```python
from build123d import *

# Parameters (mm, degrees)
BOSS_EXTRUDE1_DEPTH = 57.15
SKETCH2_W           = 44.45
SKETCH2_H           = 66.04
CUT_EXTRUDE1_DEPTH  = 57.15
SKETCH6_R           = 4.7625
CUT_EXTRUDE3_DEPTH  = 3.175
SKETCH8_R           = 0.79375
CUT_EXTRUDE4_DEPTH  = 58.15


with BuildPart() as part:
    # Sketch1 → Boss-Extrude1 (new body)
    with BuildSketch(Plane.XY):
        with BuildLine():
            Line((-15.24, 76.2), (-15.24, -76.2))
            ThreePointArc((-15.24, -76.2), (0, -91.44), (15.24, -76.2))
            Line((15.24, -76.2), (15.24, 76.2))
            ThreePointArc((15.24, 76.2), (0, 91.44), (-15.24, 76.2))
        make_face()
    extrude(amount=BOSS_EXTRUDE1_DEPTH)

    # Sketch2 → Cut-Extrude1 (cut)
    with BuildSketch(Plane(origin=(15.24, 0, 0), x_dir=(0, 0, -1), z_dir=(1, 0, 0))):
        with Locations((-28.575, 58.42)):
            Rectangle(SKETCH2_W, SKETCH2_H)
    cut_extrude1 = extrude(amount=-CUT_EXTRUDE1_DEPTH, mode=Mode.SUBTRACT)

    # Sketch6 → Cut-Extrude3 (cut)
    with BuildSketch(Plane.XY.offset(6.35)):
        with Locations((0, 76.2)):
            Circle(SKETCH6_R)
    cut_extrude3 = extrude(amount=-CUT_EXTRUDE3_DEPTH, mode=Mode.SUBTRACT)

    # Mirror3: Cut-Extrude3 across plane
    add(cut_extrude3.mirror(Plane.XY.offset(28.575)), mode=Mode.SUBTRACT)

    # Sketch8 → Cut-Extrude4 (cut, through all)
    with BuildSketch(Plane(origin=(0, 0, 0), x_dir=(-1, 0, 0), z_dir=(0, 0, -1))):
        with Locations((0, 65.88125)):
            Circle(SKETCH8_R)
        with Locations((-10.31875, 76.2)):
            Circle(SKETCH8_R)
        with Locations((0, 86.51875)):
            Circle(SKETCH8_R)
        with Locations((10.31875, 76.2)):
            Circle(SKETCH8_R)
    cut_extrude4 = extrude(amount=-CUT_EXTRUDE4_DEPTH, mode=Mode.SUBTRACT)

    # Mirror7: Cut-Extrude1, Cut-Extrude3, Cut-Extrude4 across plane
    add(cut_extrude1.mirror(Plane.ZX), mode=Mode.SUBTRACT)
    add(cut_extrude3.mirror(Plane.ZX), mode=Mode.SUBTRACT)
    add(cut_extrude4.mirror(Plane.ZX), mode=Mode.SUBTRACT)


solid = part.part
```
Part model, mm, in its own coordinate system. A direction names the side the tool comes from. Round coordinates to 2 decimals unless told otherwise and drop trailing zeros. Loops run counter-clockwise (first coordinate to the right, second up) from the corner with the lowest first, then second, coordinate; pieces in that order, holes last. Notation, with made-up numbers: (40, -17.5) -> (68, -17.5) arc R22 cw to (68, -11.5) -> close; hole circle Ø9 at (20.5, 2). An arc over 180 degrees is marked (long way). Use one line per item in the form item = value. Start each with the question number.
Item 1: Band-saw the part on A-A (y = -49). List the corners of the cut face in (x, z).
Item 2: Band-saw the part on B-B (x = -6.5). List the corners of the cut face in (y, z), plus the area to 3 significant figures.
Item 3: Band-saw the part on C-C (z = 9). List the corners of the cut face in (x, y), plus the area to 3 significant figures.
Item 4: Drill centre lines: line 1 along Y through (x, z) = (0, 53.05) (1 decimal); line 2 along X through (y, z) = (76, 4); line 3 along Y through (x, z) = (0, 2) (1 decimal). Where is each one in solid material? Low to high.
Item 5: Two-plate mould, pull along Y, no slides. Class faces 1 (the flat face through (0, 58, 50.8)), 2 (the cylindrical face through (0.335, 91.436, 3.131)), 3 (the flat face through (0, 76, 3.175)), 4 (the flat face through (0, 76, 53.975)): released by +Y, released by -Y, zero draft, split by the parting line, or undercut.
Item 6: Tool access for faces 5 (the flat face through (0, -25.4, 29)), 6 (the flat face through (0, 1, 0)), 7 (the cylindrical face through (0.335, 91.436, 53.931)), 8 (the cylindrical face through (-0.62, 80.92, 4.78)), 9 (the flat face through (0, 58, 6.35)): list every direction of +Z, -Z, +X, -X, +Y, -Y with a clear straight run to the whole face (end or side of a thin tool).
Item 7: Drop flat-ended pins along their axis: pin 1 Ø1 at (x, y) = (-3, -50.5) entering from -Z; pin 2 Ø12 at (x, z) = (-2.5, 41) entering from -Y; pin 3 Ø3 at (x, z) = (9, 17) entering from +Y. Give the stop position or say it passes through.
Data:
q1.outline = (-15.24, 0) -> (15.24, 0) -> (15.24, 6.35) -> (-15.24, 6.35) -> close; (-15.24, 50.8) -> (15.24, 50.8) -> (15.24, 57.15) -> (-15.24, 57.15) -> close
q2.outline = (-89.98, 0) -> (89.98, 0) -> (89.98, 6.35) -> (25.4, 6.35) -> (25.4, 50.8) -> (89.98, 50.8) -> (89.98, 57.15) -> (-89.98, 57.15) -> (-89.98, 50.8) -> (-25.4, 50.8) -> (-25.4, 6.35) -> (-89.98, 6.35) -> close
q2.area = 4,540 mm^2
q3.outline = (-15.24, -25.4) -> (15.24, -25.4) -> (15.24, 25.4) -> (-15.24, 25.4) -> close
q3.area = 1,550 mm^2
q4.line_1 = -91.4 to -87.3, -85.7 to -66.7, -65.1 to 65.1, 66.7 to 71.4, 81 to 85.7, 87.3 to 91.4
q4.line_2 = -15.24 to -11.09, -9.55 to -4.76, 4.76 to 9.55, 11.09 to 15.24
q4.line_3 = -91.4 to -87.3, -85.7 to -66.7, -65.1 to 65.1, 66.7 to 85.7, 87.3 to 91.4
q5.face_1 = zero draft
q5.face_2 = released by +Y
q5.face_3 = undercut
q5.face_4 = undercut
q6.face_5 = +X, -X, -Y
q6.face_6 = -Z, +X, -X, +Y, -Y
q6.face_7 = +Z, -Z, +Y
q6.face_8 = none
q6.face_9 = +X, -X, +Y
q7.pin_1 = 0
q7.pin_2 = -25.4
q7.pin_3 = 25.4
